Verification items for this drawing (mm, ordinates from the low corner). A direction names the side the tool comes from. Round coordinates to 2 decimals unless told otherwise and drop trailing zeros. Loops run counter-clockwise (first coordinate to the right, second up) from the corner with the lowest first, then second, coordinate; pieces in that order, holes last. Notation, with made-up numbers: M -38.5,54.25 L -25.5,54.25 A7 cw -25.5,64.25 Z; hole C 35,9 d6. An arc over 180 degrees is marked long. Write item = value, one per line.
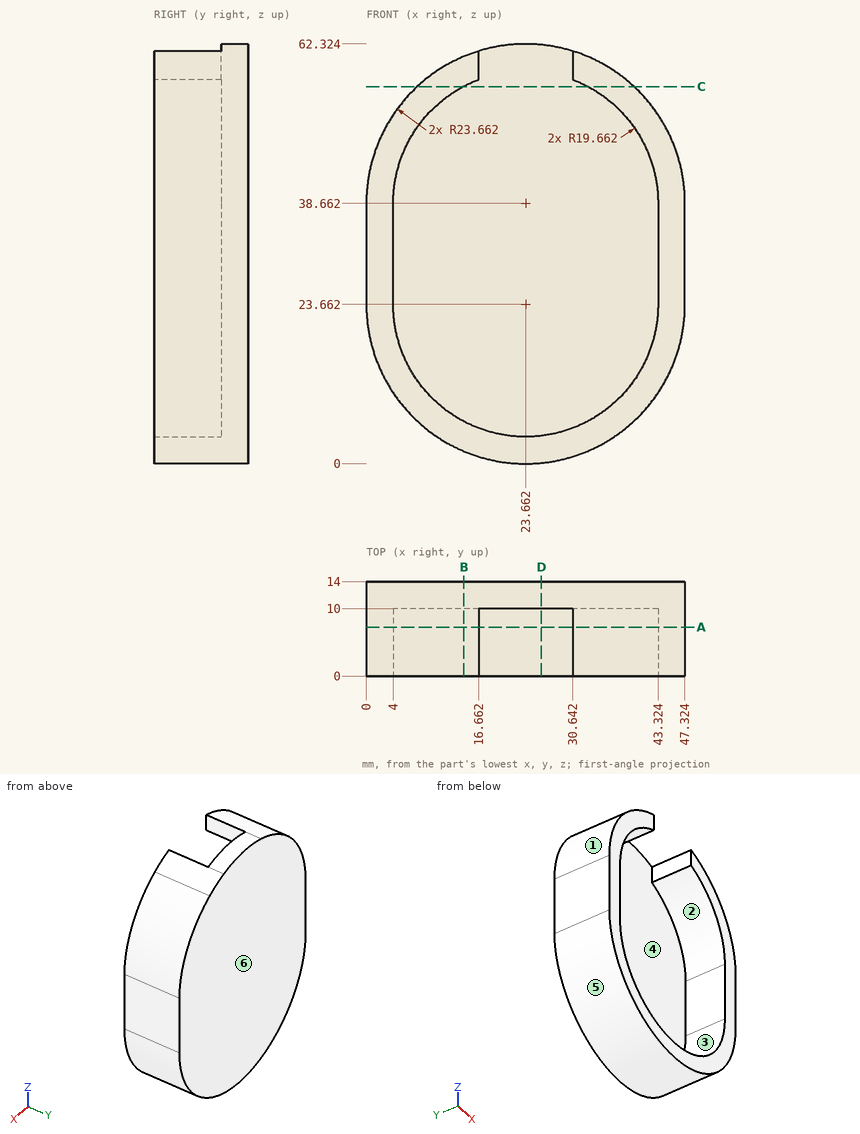
(1) Release check for a two-part mould opening along Z. For the marked faces 3, 4, 5 and 6 record: released by +Z, released by -Z, zero draft, split by the parting line, or undercut.
Result set:
face_3 = undercut
face_4 = undercut
face_5 = released by -Z
face_6 = zero draft
(2) Depth check by flat-ended pin: pin 1 Ø8 at (x, y) = (17, 6) entering from -Z; pin 2 Ø4 at (y, z) = (9.5, 10.5) entering from +X; pin 3 Ø1.3 at (y, z) = (3, 58.5) entering from +X. Enter the tip coordinate at first touch or a pass-through.
Result set:
pin_1 = 0.15
pin_2 = 44.53
pin_3 = 37.51
(3) Sectioned sample at C-C on z = 56. Record the cut outline in (x, y), then the cut area to 3 significant figures.
Result set:
outline = M 7.56,0 L 14.39,0 L 14.39,10 L 32.93,10 L 32.93,0 L 39.76,0 L 39.76,14 L 7.56,14 Z
area = 265 mm2
(4) Sectioned sample at D-D on x = 26. Record the cut outline in (y, z).
Result set:
outline = M 0,0.12 L 14,0.12 L 14,62.21 L 10,62.21 L 10,4.14 L 0,4.14 Z
(5) Material ranges on line 1 along Y through (x, z) = (34, 12); line 2 along X through (y, z) = (3, 6) (1 decimal); line 3 along Z through (x, y) = (35, 3) (1 decimal), recorded low to high. Write a range as from..to.
Result set:
line_1 = 10..14
line_2 = 7.9..15, 32.3..39.4
line_3 = 2.9..7.6, 54.7..59.4
(6) Sectioned sample at B-B on x = 14.5. Record the cut outline in (y, z) (1 decimal).
Result set:
outline = M 0,1.8 L 14,1.8 L 14,60.5 L 0,60.5 L 0,56.1 L 10,56.1 L 10,6.3 L 0,6.3 Z
(7) Tool access check on the marked faces 1 and 2. Record the directions out of +Z, -Z, +X, -X, +Y, -Y that give a thin tool (end or side, any length) a straight path to the whole face; none if there is none.
Result set:
face_1 = +Z, -X, +Y, -Y
face_2 = -Y
(8) Sectioned sample at A-A on y = 7.25. Record the cut outline in (x, z) (1 decimal).
Result set:
outline = M 0,23.7 A23.7 ccw 47.3,23.7 L 47.3,38.7 A23.7 ccw 35.9,58.9 A23.7 ccw 30.6,61.3 L 30.6,57 A19.7 cw 43.3,38.7 L 43.3,23.7 A19.7 cw 4,23.7 L 4,38.7 A19.7 cw 16.7,57 L 16.7,61.3 A23.7 ccw 0,38.7 Z
